Geometry check sheet. Reference: the model listing, model coordinates, mm. A direction names the side the tool comes from. Give positions to 0.01 mm unless a question says otherwise; leave off trailing zeros. Loops run counter-clockwise (first coordinate to the right, second up) from the corner with the lowest first, then second, coordinate; pieces in that order, holes last.
```python
from build123d import *

# Parameters (mm, degrees)
SKETCH1_R           = 18.5
BOSS_EXTRUDE1_DEPTH = 24.892
SKETCH2_R           = 18.1
BOSS_EXTRUDE2_DEPTH = 33.33
SKETCH3_R           = 6
BOSS_EXTRUDE3_DEPTH = 5
BOSS_EXTRUDE4_DEPTH = 14
SKETCH5_R           = 1.45
CUT_EXTRUDE1_DEPTH  = 5


with BuildPart() as part:
    # Sketch1 → Boss-Extrude1 (new body)
    with BuildSketch(Plane.XY):
        Circle(SKETCH1_R)
    extrude(amount=BOSS_EXTRUDE1_DEPTH)

    # Sketch2 → Boss-Extrude2 (add)
    with BuildSketch(Plane(origin=(0, 0, 0), x_dir=(-1, 0, 0), z_dir=(0, 0, -1))):
        Circle(SKETCH2_R)
    extrude(amount=BOSS_EXTRUDE2_DEPTH)

    # Sketch3 → Boss-Extrude3 (add)
    with BuildSketch(Plane.XY.offset(24.892)):
        with Locations((0, 7)):
            Circle(SKETCH3_R)
    extrude(amount=BOSS_EXTRUDE3_DEPTH)

    # Sketch4 → Boss-Extrude4 (add)
    with BuildSketch(Plane.XY.offset(29.892)):
        with BuildLine():
            Line((1.658312395, 9.5), (-1.658312395, 9.5))
            ThreePointArc((-1.658312395, 9.5), (0, 4), (1.658312395, 9.5))
        make_face()
    extrude(amount=BOSS_EXTRUDE4_DEPTH)

    # Sketch5 → Cut-Extrude1 (cut)
    with BuildSketch(Plane.XY.offset(24.892)):
        with Locations((15.5, 0)):
            Circle(SKETCH5_R)
        with Locations((7.75, -13.423393759)):
            Circle(SKETCH5_R)
        with Locations((-7.75, -13.423393759)):
            Circle(SKETCH5_R)
        with Locations((-15.5, 0)):
            Circle(SKETCH5_R)
        with Locations((-7.75, 13.423393759)):
            Circle(SKETCH5_R)
        with Locations((7.75, 13.423393759)):
            Circle(SKETCH5_R)
    extrude(amount=-CUT_EXTRUDE1_DEPTH, mode=Mode.SUBTRACT)


solid = part.part
```
1) Tool access check on faces 5 (the cylindrical face through (-14.12, 0.44, 22.43)), 6 (the flat face through (0, 7, 43.892)). Record the directions out of +Z, -Z, +X, -X, +Y, -Y that give a thin tool (end or side, any length) a straight path to the whole face; none if there is none.
2) Sectioned sample at C-C on z = 28. Enter the section's corners in (x, y).
3) Sectioned sample at A-A on y = 0. Enter the section's corners in (x, z), plus the area to 3 significant figures.
4) Sectioned sample at D-D on x = -15.5. Enter the section's corners in (y, z).
5) Mould release check, pull along Y, two halves, no side actions. Record for faces 1 (the flat face through (13.6, -12.2, 0)), 2 (the flat face through (-8, 13, 19.892)), 3 (the flat face through (0, 9.5, 37)), 4 (the cylindrical face through (-8.9, 12.54, 22.43)): +Y half, -Y half, draft (parallel to the pull), parting line (faces both ways), or undercut.
6) Sectioned sample at B-B on x = 0. Enter the section's corners in (y, z).
7) Depth check by flat-ended pin: P1, Ø6, axis at x = -2, y = -10.5, coming from the +Z side; P2, Ø0.9, axis at x = 15, y = 0.5, coming from the +Z side; P3, Ø10, axis at y = 6.5, z = 36, coming from the +X side. Enter the tip coordinate at first touch or a pass-through.
8) Scan lines: line 1 along Y through (x, z) = (-7.75, 22.3); line 2 along Y through (x, z) = (-7, 22); line 3 along Z through (x, y) = (-12.5, -11). Record each from-to range of solid material in increasing order.
Determined:
1. face 5: +Z
1. face 6: +Z, +X, -X, +Y, -Y
2. outline: circle Ø12 at (0, 7)
3. outline: (-18.5, 0) - (-18.1, 0) - (-18.1, -33.33) - (18.1, -33.33) - (18.1, 0) - (18.5, 0) - (18.5, 24.89) - (16.95, 24.89) - (16.95, 19.89) - (14.05, 19.89) - (14.05, 24.89) - (-14.05, 24.89) - (-14.05, 19.89) - (-16.95, 19.89) - (-16.95, 24.89) - (-18.5, 24.89) - close
3. area: 2,100 mm2
4. outline: (-10.1, 0) - (-9.35, 0) - (-9.35, -33.33) - (9.35, -33.33) - (9.35, 0) - (10.1, 0) - (10.1, 24.89) - (1.45, 24.89) - (1.45, 19.89) - (-1.45, 19.89) - (-1.45, 24.89) - (-10.1, 24.89) - close
5. face 1: draft
5. face 2: undercut
5. face 3: +Y half
5. face 4: undercut
6. outline: (-18.5, 0) - (-18.1, 0) - (-18.1, -33.33) - (18.1, -33.33) - (18.1, 0) - (18.5, 0) - (18.5, 24.89) - (13, 24.89) - (13, 29.89) - (9.5, 29.89) - (9.5, 43.89) - (4, 43.89) - (4, 29.89) - (1, 29.89) - (1, 24.89) - (-18.5, 24.89) - close
7. P1: stops at z = 24.89
7. P2: stops at z = 19.89
7. P3: stops at x = 3
8. line 1: y = -16.8 to -14.87, -11.97 to 11.97, 14.87 to 16.8
8. line 2: y = -17.12 to -14.66, -12.18 to 12.18, 14.66 to 17.12
8. line 3: z = -33.33 to 24.89
